Geometry check sheet. Reference: the model listing, model coordinates, mm. A direction names the side the tool comes from. Round coordinates to 2 decimals unless told otherwise and drop trailing zeros. Order: outer loops, then holes, each group sorted by start corner. A loop starts at its lowest first (then second) coordinate and runs counter-clockwise, first axis right, second up. Notation, with made-up numbers: (21, 8) -> (42, 8) arc R24 ccw to (42, 38) -> close; hole circle Ø6 at (64.25, 59.5). An arc over 180 degrees is marked (long way). Use a Markdown table: item, result. Add a question column.
Item 1: Material ranges on probe 1 along Z at (x, y) = (0.4, 12.7) (3 decimals); probe 2 along X at (y, z) = (13.5, -23), recorded low to high. Write a range as [from, to].
Item 2: Sectioned sample at B-B, the plane z = -135. Record the cut outline in (x, y), and give its area (3 significant figures).
Item 3: Sectioned sample at A-A, the plane y = 12.7. Record the cut outline in (x, z) (1 decimal).
Item 4: Set-up check for faces 1 (the flat face through (13, 23.812, -88)), 2 (the cylindrical face through (24.62, 13.92, -162.17)): record each of +Z, -Z, +X, -X, +Y, -Y from which the full face is reachable in a straight line by a thin tool's end or side.
Item 5: Mould release check, pull along X, two halves, no side actions. Record for faces 3 (the flat face through (25.4, 13, -88)), 4 (the cylindrical face through (14.63, 24.62, -10.18)), 5 (the flat face through (1, 13, -177.8)), 6 (the flat face through (0, 13, -88)): pulls with the +X half, pulls with the -X half, needs draft (parallel to the pull), parting line crosses it, or undercut.
Item 6: Sectioned sample at C-C, the plane y = 4. Record the cut outline in (x, z).
Autodesk Inventor part; units mm, degrees
ref_plane "YZ Plane" through (0, 0, 0) normal (1, 0, 0) x (0, 1, 0)
ref_plane "XZ Plane" through (0, 0, 0) normal (0, 1, 0) x (-1, 0, 0)
ref_plane "XY Plane" through (0, 0, 0) normal (0, 0, 1) x (1, 0, 0)
sketch "Sketch1" plane through (0, 0, 0) normal (0, 0, 1) x (1, 0, 0)
  line L0 (0, 0) -> (25.4, 0)
  line L1 (25.4, 0) -> (25.4, 25.4)
  line L2 (25.4, 25.4) -> (0, 25.4)
  line L3 (0, 25.4) -> (0, 0)
  line L4 (1.5875, 23.8125) -> (23.8125, 23.8125)
  line L5 (23.8125, 23.8125) -> (23.8125, 1.5875)
  line L6 (23.8125, 1.5875) -> (1.5875, 1.5875)
  line L7 (1.5875, 1.5875) -> (1.5875, 23.8125)
  dimension "d0" = 25.4
  dimension "d1" = 25.4
  dimension "d2" = 1.5875
extrude "Extrusion1" add sketch "Sketch1" against normal blind 177.8
sketch "Sketch2" plane through (0, 0, 0) normal (0, -1, 0) x (1, 0, 0)
  line L0 (0, -177.8) -> (25.4, -177.8)
  line L1 (0, 0) -> (25.4, 0)
  point P0 (12.7, -12.7)
  point P1 (12.7, -165.1)
  dimension "d5" = 12.7
  dimension "d6" = 12.7
hole "Hole1" at (12.7, 0, -12.7) at (12.7, 0, -165.1) direction (0, 1, 0) diameter 6.35 depth 25.4 tip angle 118
sketch "Sketch3" plane through (0, 0, 0) normal (-1, 0, 0) x (0, 0, 1)
  line L0 (-177.8, 25.4) -> (-177.8, 0)
  line L1 (0, 25.4) -> (0, 0)
  point P0 (-12.7, 12.7)
  point P1 (-165.1, 12.7)
  dimension "d14" = 12.7
  dimension "d15" = 12.7
hole "Hole2" at (0, 12.7, -12.7) at (0, 12.7, -165.1) direction (1, 0, 0) diameter 6.35 depth 25.4 tip angle 118
properties part number "1tube_6_layer1_motorsupport"
Found:
| question | item | result |
|---|---|---|
| 1 | probe 1 | z = [-177.8, -168.275], [-161.925, -15.875], [-9.525, 0] |
| 1 | probe 2 | x = [0, 1.59], [23.81, 25.4] |
| 2 | outline | (0, 0) -> (25.4, 0) -> (25.4, 25.4) -> (0, 25.4) -> close; hole (1.59, 1.59) -> (23.81, 1.59) -> (23.81, 23.81) -> (1.59, 23.81) -> close |
| 2 | area | 151 mm2 |
| 3 | outline | (0, -177.8) -> (1.6, -177.8) -> (1.6, -168.3) -> (0, -168.3) -> close; (0, -161.9) -> (1.6, -161.9) -> (1.6, -15.9) -> (0, -15.9) -> close; (0, -9.5) -> (1.6, -9.5) -> (1.6, 0) -> (0, 0) -> close; (23.8, -177.8) -> (25.4, -177.8) -> (25.4, -168.3) -> (23.8, -168.3) -> close; (23.8, -161.9) -> (25.4, -161.9) -> (25.4, -15.9) -> (23.8, -15.9) -> close; (23.8, -9.5) -> (25.4, -9.5) -> (25.4, 0) -> (23.8, 0) -> close |
| 4 | face 1 | +Z, -Z |
| 4 | face 2 | +X, -X |
| 5 | face 3 | pulls with the +X half |
| 5 | face 4 | undercut |
| 5 | face 5 | needs draft |
| 5 | face 6 | pulls with the -X half |
| 6 | outline | (0, -177.8) -> (1.59, -177.8) -> (1.59, 0) -> (0, 0) -> close; (23.81, -177.8) -> (25.4, -177.8) -> (25.4, 0) -> (23.81, 0) -> close |
